from build123d import *

# Parameters (mm, degrees)
F1_DEPTH = 1.397
F2_R     = 4.1402
F3_R     = 1.397


with BuildPart() as f1:
    # F0 (on Top) → F1 (new body)
    with BuildSketch(Plane.XY):
        Polygon((-97.091727, 139.401406), (-153.911527, 139.401406), (-149.916979, 109.059797), (-168.39164, 99.442497), (-148.55581, -51.225594), (0, -51.225594), (147.53981, -51.225594), (167.37564, 99.442497), (148.900979, 109.059797), (152.895527, 139.401406), (96.075727, 139.401406), (96.896243, 144.631802), (0, 151.339406), (-97.906282, 144.544299), align=None)
        Polygon((-131.826, -39.033594), (-131.826, 124.796406), (0, 124.796406), (130.81, 124.796406), (131.826, 124.796406), (131.826, -39.033594), (-1.016, -39.033594), align=None, mode=Mode.SUBTRACT)
    extrude(amount=F1_DEPTH)

    # F2
    f2_edges = [f1.edges().sort_by_distance(p)[0] for p in [
        (-153.911527, 139.401406, 0.6985),
        (152.895527, 139.401406, 0.6985),
        (-168.39164, 99.442497, 0.6985),
        (167.37564, 99.442497, 0.6985),
    ]]
    fillet(f2_edges, radius=F2_R)

    # F3
    f3_edges = [f1.edges().sort_by_distance(p)[0] for p in [
        (96.896243, 144.631802, 0.6985),
        (-97.906282, 144.544299, 0.6985),
    ]]
    fillet(f3_edges, radius=F3_R)


solid = f1.part
Design review of the part built by this model. Coordinates are the model's own, in mm. A direction names the side the tool comes from. Coordinates: 2 decimals unless noted, no trailing zeros. Loops run counter-clockwise (first coordinate to the right, second up) from the corner with the lowest first, then second, coordinate; pieces in that order, holes last. Notation, with made-up numbers: M -26.5,-9.5 L 7.5,-9.5 A25 cw 7.5,16.5 Z; hole C 45,-15.75 d1. An arc over 180 degrees is marked long. Use one line per item in the form item = value.
(1) For faces 4 (the face through (11, 126, 0)), 5 (the face through (-157.757, 104.978, 0.689)), list the 3-axis set-ups (+Z, -Z, +X, -X, +Y, -Y) from which the entire face can be reached by the end or side of a thin tool; tool diameter is ignored.
Return value:
face_4 = -Z, +X, -X, +Y, -Y
face_5 = +Z, -Z, -X
(2) Consider section A-A (z = 0.8). Write out the cut boundary in (x, y).
Return value:
outline = M -168.01,96.57 L -148.56,-51.23 L 147.54,-51.23 L 167,96.57 A4.14 ccw 164.8,100.78 L 148.9,109.06 L 152.28,134.72 A4.14 ccw 148.17,139.4 L 96.08,139.4 L 96.66,143.13 A1.4 ccw 95.38,144.74 L 0,151.34 L -96.38,144.65 A1.4 ccw -97.67,143.04 L -97.09,139.4 L -149.19,139.4 A4.14 ccw -153.3,134.72 L -149.92,109.06 L -165.82,100.78 A4.14 ccw Z; hole M -131.83,-39.03 L 131.83,-39.03 L 131.83,124.8 L -131.83,124.8 Z
(3) Consider section B-B (y = 62). Write out the cut boundary in (x, z), and give its area (3 significant figures).
Return value:
outline = M -163.46,0 L -131.83,0 L -131.83,1.4 L -163.46,1.4 Z; M 131.83,0 L 162.45,0 L 162.45,1.4 L 131.83,1.4 Z
area = 87.0 mm2
(4) For line 1 along Y through (x, z) = (-96, 1.15); line 2 along Y through (x, z) = (122, 0.95); line 3 along X through (y, z) = (30.5, 1.2), list the stretches that pass through material, from the lowest coordinate up. Write a range as from..to.
Return value:
line_1 = -51.23..-39.03, 124.8..144.68
line_2 = -51.23..-39.03, 124.8..139.4
line_3 = -159.32..-131.83, 131.83..158.3
(5) Clearance check with flat-ended pins moving along their axes: P1, Ø6, axis at x = -41.5, y = 122.5, coming from the -Z side; P2, Ø0.7, axis at x = 127.5, z = 0.5, coming from the +Y side; P3, Ø0.7, axis at y = 49.5, z = 1, coming from the +X side; P4, Ø8, axis at x = 59, y = 118.5, coming from the +Z side. State where each tip first meets the part, or that it passes through.
Return value:
P1 = 0
P2 = 139.4
P3 = 160.85
P4 = through
(6) Consider section C-C (x = 82). Write out the cut boundary in (y, z).
Return value:
outline = M -51.23,0 L -39.03,0 L -39.03,1.4 L -51.23,1.4 Z; M 124.8,0 L 145.66,0 L 145.66,1.4 L 124.8,1.4 Z
(7) Draft analysis for pull direction Y (two halves, no side actions). For faces 1 (the face through (156.964, 104.863, 0.689)), 2 (the face through (-158.42, 23.71, 0.69)), 3 (the face through (-47.52, 148.04, 0.69)), state which applies: pulls with the +Y half, pulls with the -Y half, needs draft (parallel to the pull), parting line crosses it, or undercut.
Return value:
face_1 = undercut
face_2 = pulls with the -Y half
face_3 = pulls with the +Y half
